Check sheet for the modelled part. Datum: model origin and axes. Units: mm. A direction names the side the tool comes from. Give positions to 0.01 mm unless a question says otherwise; leave off trailing zeros. Order: outer loops, then holes, each group sorted by start corner. A loop starts at its lowest first (then second) coordinate and runs counter-clockwise, first axis right, second up.
Item 1: Sectioned sample at B-B on x = 6. Record the boundary of the cut face in (y, z), and give its area (3 significant figures).
Item 2: Gauge pin test, flat ends, axial feed: P1, Ø12, axis at x = 32, z = -2.5, coming from the +Y side; P2, Ø0.6, axis at y = 11.5, z = 4.5, coming from the +X side; P3, Ø5, axis at x = 22, z = -8.5, coming from the -Y side; P4, Ø10, axis at x = 29, y = 12.5, coming from the -Z side. Record the tip position at first contact, or that the pin passes through.
Item 3: Access from +Z, -Z, +X, -X, +Y, -Y to the whole of each face (thin tool, end or side, straight path). Record for faces 1 (the flat face through (33, 7, 3)), 2 (the flat face through (33, 7, -3)), 3 (the flat face through (46.388, 2, 0)), 4 (the flat face through (5, 19, -2)).
Item 4: Sectioned sample at C-C on z = -1.25. Record the boundary of the cut face in (x, y).
Item 5: Sectioned sample at D-D on y = 7.75. Record the boundary of the cut face in (x, z), and give its area (3 significant figures).
Item 6: Material ranges on line 1 along Z through (x, y) = (47, 15.5); line 2 along Z through (x, y) = (20.5, 11.25); line 3 along X through (y, z) = (3.25, 6), recorded low to high.
Item 7: Release check for a two-part mould opening along X. For faces 5 (the flat face through (44, 10, -4)), 6 (the flat face through (8, 16, 0)), 7 (the flat face through (0, 11, 0)) record: released by +X, released by -X, zero draft, split by the parting line, or undercut.
Item 8: Sectioned sample at A-A on y = 3.75. Record the boundary of the cut face in (x, z).
from build123d import *

# Parameters (mm, degrees)
SKETCH_1_W           = 25
SKETCH_1_H           = 4.8
EXTRUDE_1_DEPTH      = 4
EXTRUDE_1_DEPTH_BACK = 4


with BuildPart() as part:
    # Sketch 1 → Revolve 1 (revolve)
    with BuildSketch(Plane.XY, mode=Mode.PRIVATE) as revolve_1_sk:
        Polygon((0, 11), (0, 0), (5, 0), (5, 3), (5, 11), align=None)
        Polygon((5, 11), (5, 3), (8, 3), (8, 6.2), (8, 11), align=None)
        with Locations((20.5, 8.6)):
            Rectangle(SKETCH_1_W, SKETCH_1_H)
    revolve(revolve_1_sk.sketch.rotate(Axis((0, 11, 0), (1, 0, 0)), 270), axis=Axis((0, 11, 0), (1, 0, 0)))

    # Sketch 1_3 → Extrude 1 (add, two sides: drawn at the far end of the back side and taken through both)
    with BuildSketch(Plane.XY.offset(-EXTRUDE_1_DEPTH_BACK)):
        Polygon((33, 15.8), (33, 6.2), (46.388094458, 6.2), (46.388094458, -1.517423247), (49.961353524, -1.517423247), (54.964630107, 11), (44.95807694, 21.414261094), align=None)
    extrude(amount=EXTRUDE_1_DEPTH + EXTRUDE_1_DEPTH_BACK)


solid = part.part
Report:
1. outline: circle Ø16 at (11, 0)
1. area: 201 mm2
2. P1: stops at y = 18.15
2. P2: stops at x = 33
2. P3: passes through
2. P4: stops at z = -4.8
3. face 1: +Z, -Y
3. face 2: -Z, -Y
3. face 3: +Z, -Z, -Y
3. face 4: none
4. outline: (0, 0.07) - (5, 0.07) - (5, 3.1) - (8, 3.1) - (8, 6.37) - (33, 6.37) - (33, 6.2) - (46.39, 6.2) - (46.39, -1.52) - (49.96, -1.52) - (54.96, 11) - (44.96, 21.41) - (33, 15.8) - (33, 15.63) - (8, 15.63) - (8, 18.9) - (5, 18.9) - (5, 21.93) - (0, 21.93) - close
5. outline: (0, -10.51) - (5, -10.51) - (5, -7.31) - (8, -7.31) - (8, -3.53) - (33, -3.53) - (33, -4) - (53.67, -4) - (53.67, 4) - (33, 4) - (33, 3.53) - (8, 3.53) - (8, 7.31) - (5, 7.31) - (5, 10.51) - (0, 10.51) - close
5. area: 491 mm2
6. line 1: z = -4 to 4
6. line 2: z = -4.79 to 4.79
6. line 3: x = 0 to 5
7. face 5: zero draft
7. face 6: undercut
7. face 7: released by -X
8. outline: (0, -8.27) - (5, -8.27) - (5, -3.38) - (8, -3.38) - (8, 3.38) - (5, 3.38) - (5, 8.27) - (0, 8.27) - close; (46.39, -4) - (52.07, -4) - (52.07, 4) - (46.39, 4) - close
